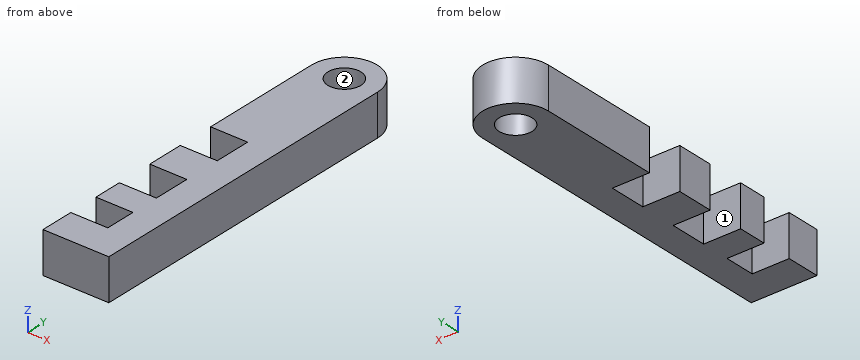
from build123d import *

# Parameters (mm, degrees)
ESQUISSE1_R        = 2
BOSS_EXTRU_1_DEPTH = 5


with BuildPart() as part:
    # Esquisse1 → Boss.-Extru.1 (new body)
    with BuildSketch(Plane.XY):
        with BuildLine():
            Line((-60.818649801, 1.004609912), (-60.818649801, 11.306245912))
            ThreePointArc((-60.818649801, 11.306245912), (-56.818649801, 15.306245912), (-52.818649801, 11.306245912))
            Line((-52.818649801, 11.306245912), (-52.818649801, -28.402433088))
            Line((-52.818649801, -28.402433088), (-60.818649801, -28.402433088))
            Line((-60.818649801, -28.402433088), (-60.818649801, -24.294096088))
            Line((-60.818649801, -24.294096088), (-56.318649801, -24.294096088))
            Line((-56.318649801, -24.294096088), (-56.318649801, -20.573332088))
            Line((-56.318649801, -20.573332088), (-60.818649801, -20.573332088))
            Line((-60.818649801, -20.573332088), (-60.818649801, -17.109221088))
            Line((-60.818649801, -17.109221088), (-56.318649801, -17.109221088))
            Line((-56.318649801, -17.109221088), (-56.318649801, -12.609221088))
            Line((-56.318649801, -12.609221088), (-60.818649801, -12.609221088))
            Line((-60.818649801, -12.609221088), (-60.818649801, -8.109221088))
            Line((-60.818649801, -8.109221088), (-56.318649801, -8.109221088))
            Line((-56.318649801, -8.109221088), (-56.318649801, -3.609221088))
            Line((-56.318649801, -3.609221088), (-60.818649801, -3.609221088))
            Line((-60.818649801, -3.609221088), (-60.818649801, 1.004609912))
        make_face()
        with Locations((-56.818649801, 11.306245912)):
            Circle(ESQUISSE1_R, mode=Mode.SUBTRACT)
    extrude(amount=BOSS_EXTRU_1_DEPTH)


solid = part.part
Work out the finished part from the listing and answer in its coordinate system (mm). Face numbers are marked on the shaded views. A direction names the side the tool comes from. Give positions to 0.01 mm unless a question says otherwise; leave off trailing zeros. Order: outer loops, then holes, each group sorted by start corner. A loop starts at its lowest first (then second) coordinate and runs counter-clockwise, first axis right, second up. Notation, with made-up numbers: (32, 48.25) -> (88, 48.25) arc R19 cw to (88, 77.25) -> close; hole circle Ø8 at (-14.75, 24.25). An arc over 180 degrees is marked (long way). Answer as a JSON object with one key per item and string values. Group by question number.
1. Consider line 1 along Y through (x, z) = (-56.75, 4.4); line 2 along Y through (x, z) = (-57.75, 2.05); line 3 along Y through (x, z) = (-59, 1.8). Determine where each line is inside the solid, lowest interval first. Write a range as [from, to].
2. A tool of negligible diameter and unlimited length cuts with its end or side. For the marked faces 1 and 2, from which of +Z, -Z, +X, -X, +Y, -Y can it reach the whole face along a straight path? Write none if from no direction.
3. Section D-D on x = -55.25 is taken. Determine the outline of the cut face in (y, z), plus the area to 3 significant figures.
4. Section C-C on x = -59.75 is taken. Determine the outline of the cut face in (y, z).
5. Section A-A on z = 2.5 is taken. Determine the outline of the cut face in (x, y).
6. Section B-B on y = 12.5 is taken. Determine the outline of the cut face in (x, z).
7. Flat-ended cylindrical pins translate along their axes: pin 1 Ø2.5 at (y, z) = (-14.5, 2) entering from -X; pin 2 Ø1.3 at (x, z) = (-59.5, 3) entering from +Y; pin 3 Ø2 at (x, z) = (-59, 1.5) entering from +Y. Find the tip coordinate at first contact, or state that the pin passes through.
Result sheet:
{
 "1": {"line 1": "y = [-28.4, -24.29], [-20.57, -17.11], [-12.61, -8.11], [-3.61, 9.31], [13.31, 15.31]", "line 2": "y = [-28.4, -24.29], [-20.57, -17.11], [-12.61, -8.11], [-3.61, 9.54], [13.08, 15.2]", "line 3": "y = [-28.4, -24.29], [-20.57, -17.11], [-12.61, -8.11], [-3.61, 14.66]"},
 "2": {"face 1": "+Z, -Z, -X", "face 2": "+Z, -Z"},
 "3": {"outline": "(-28.4, 0) -> (10.07, 0) -> (10.07, 5) -> (-28.4, 5) -> close; (12.55, 0) -> (14.99, 0) -> (14.99, 5) -> (12.55, 5) -> close", "area": "205 mm^2"},
 "4": {"outline": "(-28.4, 0) -> (-24.29, 0) -> (-24.29, 5) -> (-28.4, 5) -> close; (-20.57, 0) -> (-17.11, 0) -> (-17.11, 5) -> (-20.57, 5) -> close; (-12.61, 0) -> (-8.11, 0) -> (-8.11, 5) -> (-12.61, 5) -> close; (-3.61, 0) -> (14.03, 0) -> (14.03, 5) -> (-3.61, 5) -> close"},
 "5": {"outline": "(-60.82, -28.4) -> (-52.82, -28.4) -> (-52.82, 11.31) arc R4 ccw to (-60.82, 11.31) -> (-60.82, -3.61) -> (-56.32, -3.61) -> (-56.32, -8.11) -> (-60.82, -8.11) -> (-60.82, -12.61) -> (-56.32, -12.61) -> (-56.32, -17.11) -> (-60.82, -17.11) -> (-60.82, -20.57) -> (-56.32, -20.57) -> (-56.32, -24.29) -> (-60.82, -24.29) -> close; hole circle Ø4 at (-56.82, 11.31)"},
 "6": {"outline": "(-60.64, 0) -> (-58.42, 0) -> (-58.42, 5) -> (-60.64, 5) -> close; (-55.21, 0) -> (-53, 0) -> (-53, 5) -> (-55.21, 5) -> close"},
 "7": {"pin 1": "stops at x = -56.32", "pin 2": "stops at y = 14.75", "pin 3": "stops at y = 15.13"}
}
